The listing builds one solid part. Answer for the finished solid, in the listing's coordinates (mm). A direction names the side the tool comes from. Round coordinates to 2 decimals unless told otherwise and drop trailing zeros. Write each loop counter-clockwise with the first axis right and the second up, starting at its lowest first coordinate (ties: lowest second). Pieces come first, ordered by that corner, then holes. Notation, with made-up numbers: M 52,67 L 81,67 A30 ccw 81,89 Z; hole C 11,30.5 d2. An arc over 180 degrees is marked long. Write each question's results on one line, items separated by ' | '.
from build123d import *

# Parameters (mm, degrees)
SKETCH_W            = 160
SKETCH_H            = 50
SKETCH_R            = 3
PAD_DEPTH           = 6
POCKET_DEPTH        = 1
POCKET001_DEPTH     = 1
LINEARPATTERN_COUNT = 30
LINEARPATTERN_PITCH = 2.224138
FILLET_R            = 5


with BuildPart() as part:
    # Sketch → Pad (new body)
    with BuildSketch(Plane.XY):
        Rectangle(SKETCH_W, SKETCH_H)
        with Locations((-75, 18)):
            Circle(SKETCH_R, mode=Mode.SUBTRACT)
        with Locations((75, 18)):
            Circle(SKETCH_R, mode=Mode.SUBTRACT)
        with Locations((75, -18)):
            Circle(SKETCH_R, mode=Mode.SUBTRACT)
        with Locations((-75, -18)):
            Circle(SKETCH_R, mode=Mode.SUBTRACT)
        with Locations((0, -18)):
            Circle(SKETCH_R, mode=Mode.SUBTRACT)
        with Locations((0, 18)):
            Circle(SKETCH_R, mode=Mode.SUBTRACT)
    extrude(amount=PAD_DEPTH)

    # Sketch001 (on Face12 of Pad) → Pocket (cut)
    with BuildSketch(Plane.XY.offset(6)):
        with BuildLine():
            Line((-70, -10), (-70, 12))
            Line((-70, 12), (0, 12))
            Line((0, 12), (0, 4))
            Line((0, 4), (-67, 4))
            Line((-67, 4), (-69.005, -10.070536))
            ThreePointArc((-70, -10), (-69.535356, -10.498748), (-69.005, -10.070536))
        make_face()
    extrude(amount=-POCKET_DEPTH, mode=Mode.SUBTRACT)

    # Sketch002 → Pocket001 (cut)
    with BuildSketch(Plane.XY.offset(6)):
        with BuildLine():
            Line((-67, 4), (-66.5, -7.521698))
            ThreePointArc((-66.5, -7.521698), (-66, -8.000471), (-65.5, -7.521698))
            Line((-65, 4), (-65.5, -7.521698))
            Line((-67, 4), (-65, 4))
        make_face()
    pocket001 = extrude(amount=-POCKET001_DEPTH, mode=Mode.SUBTRACT)

    # LinearPattern: Pocket001 ×30
    with Locations(*[(i * LINEARPATTERN_PITCH, 0, 0) for i in range(1, LINEARPATTERN_COUNT)]):
        add(pocket001, mode=Mode.SUBTRACT)

    # Fillet
    fillet_edges = [part.edges().sort_by_distance(p)[0] for p in [
        (-70, 12, 5.5),
    ]]
    fillet(fillet_edges, radius=FILLET_R)


solid = part.part
1) Section C-C (z = 2.75) is taken. Determine the outline of the cut face in (x, y), then the cut area to 3 significant figures.
Return value:
outline: M -80,-25 L 80,-25 L 80,25 L -80,25 Z; hole C -75,-18 d6; hole C -75,18 d6; hole C 0,-18 d6; hole C 0,18 d6; hole C 75,-18 d6; hole C 75,18 d6 | area: 7,830 mm²
2) The mould has two halves that part along Y. Classify faces 3 (the face through (-35, 3, 5)), 4 (the face through (-1, -25, 3)), 5 (the face through (17, 0, 6)), 6 (the face through (-1, 25, 3)): +Y half, -Y half, draft (parallel to the pull), parting line (faces both ways), or undercut.
Return value:
face 3: undercut | face 4: -Y half | face 5: draft | face 6: +Y half
3) This flat-tipped pin is pushed along its axis until it touches: pin 1 (5 mm diameter, centred on x = 44.5, y = -11, fed in from -Z). Where does it stop, or does it pass through?
Return value:
pin 1: z = 0
4) Section B-B (x = 75) is taken. Determine the outline of the cut face in (y, z).
Return value:
outline: M -25,0 L -21,0 L -21,6 L -25,6 Z; M -15,0 L 15,0 L 15,6 L -15,6 Z; M 21,0 L 25,0 L 25,6 L 21,6 Z
5) Section A-A (y = 18) is taken. Determine the outline of the cut face in (x, z), then the cut area to 3 significant figures.
Return value:
outline: M -80,0 L -78,0 L -78,6 L -80,6 Z; M -72,0 L -3,0 L -3,6 L -72,6 Z; M 3,0 L 72,0 L 72,6 L 3,6 Z; M 78,0 L 80,0 L 80,6 L 78,6 Z | area: 852 mm²
6) Find the intervals of material crossed by line 1 (Y direction, x = 75, z = 2.8); line 2 (X direction, y = -10, z = 5.15); line 3 (Y direction, x = -33, z = 5.1), in increasing order.
Return value:
line 1: -25 to -21, -15 to 15, 21 to 25 | line 2: -80 to -70, -68.99 to 80 | line 3: -25 to -7.85, 12 to 25
7) A tool of negligible diameter and unlimited length cuts with its end or side. For faces 1 (the face through (-68.5, 10.57, 5.49)), 2 (the face through (-77.4, 16.2, 3)), from which of +Z, -Z, +X, -X, +Y, -Y can it reach the whole face along a straight path? Write none if from no direction.
Return value:
face 1: +Z | face 2: +Z, -Z
